from build123d import *

# Parameters (mm, degrees)
SKETCH_1_W               = 9.9
SKETCH_1_H               = 65.9
EXTRUDE_1_DEPTH          = 2
SKETCH_2_R               = 1.6
CUT_EXTRUDE_1_DEPTH      = 1
CUT_EXTRUDE_1_DEPTH_BACK = 3


with BuildPart() as part:
    # Эскиз1 → Бобышка-Вытянуть1 (new body)
    with BuildSketch(Plane(origin=(0, 0, 0), x_dir=(1, 0, 0), z_dir=(0, 1, 0))):
        Rectangle(SKETCH_1_W, SKETCH_1_H)
    extrude(amount=EXTRUDE_1_DEPTH)

    # Эскиз2 → Вырез-Вытянуть1 (cut, two sides)
    with BuildSketch(Plane(origin=(0, 2, 0), x_dir=(1, 0, 0), z_dir=(0, 1, 0))) as cut_extrude_1_sk:
        with Locations((1.95, 20)):
            Circle(SKETCH_2_R)
        with Locations((1.95, -20)):
            Circle(SKETCH_2_R)
    extrude(amount=CUT_EXTRUDE_1_DEPTH, mode=Mode.SUBTRACT)
    extrude(cut_extrude_1_sk.sketch, amount=-CUT_EXTRUDE_1_DEPTH_BACK, mode=Mode.SUBTRACT)


solid = part.part
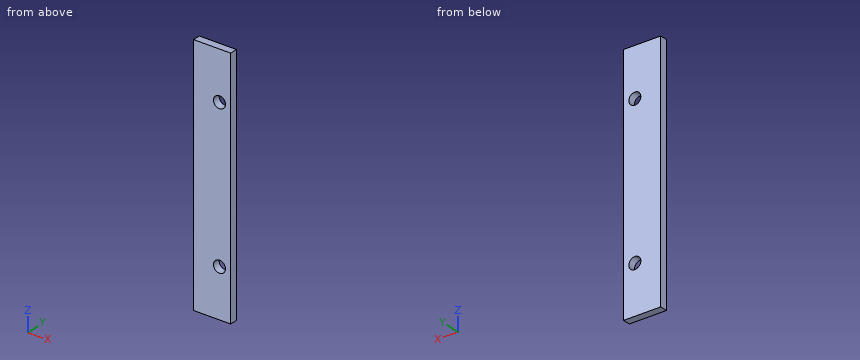
Part model, mm, in its own coordinate system. Coordinates: 2 decimals unless noted, no trailing zeros. Order: outer loops, then holes, each group sorted by start corner. A loop starts at its lowest first (then second) coordinate and runs counter-clockwise, first axis right, second up. Notation, with made-up numbers: M -21.75,83.5 L -14.75,83.5 A25 ccw -14.75,122.5 Z; hole C 40.25,39 d8. An arc over 180 degrees is marked long. One line per question, with ' | ' between items.
Q1. Slice it at B-B (x = 1.95). Give the cut face in (y, z).
A:
outline: M 0,-32.95 L 2,-32.95 L 2,-21.6 L 0,-21.6 Z; M 0,-18.4 L 2,-18.4 L 2,18.4 L 0,18.4 Z; M 0,21.6 L 2,21.6 L 2,32.95 L 0,32.95 Z
Q2. Drill centre lines: line 1 (Z direction, x = 1.95, y = 0.8); line 2 (X direction, y = 1.3, z = 20); line 3 (Z direction, x = 1.5, y = 1.2). Where is each one in solid material? Low to high.
A:
line 1: z = -32.95 to -21.6, -18.4 to 18.4, 21.6 to 32.95 | line 2: x = -4.95 to 0.35, 3.55 to 4.95 | line 3: z = -32.95 to -21.54, -18.46 to 18.46, 21.54 to 32.95
Q3. Slice it at A-A (z = 20). Give the cut face in (x, y), and give its area (3 significant figures).
A:
outline: M -4.95,0 L 0.35,0 L 0.35,2 L -4.95,2 Z; M 3.55,0 L 4.95,0 L 4.95,2 L 3.55,2 Z | area: 13.4 mm^2
Q4. Pin check, flat tip, straight feed: P1, Ø3, axis at x = 1.95, z = -20, coming from the -Y side. Stop position of the tip, or through.
A:
P1: passes through
Q5. Slice it at C-C (y = 1.2). Give the cut face in (x, z), and give its area (3 significant figures).
A:
outline: M -4.95,-32.95 L 4.95,-32.95 L 4.95,32.95 L -4.95,32.95 Z; hole C 1.95,-20 d3.2; hole C 1.95,20 d3.2 | area: 636 mm^2
